Read the model definition and answer for the solid it produces. Units are mm, in the model's axes. Face numbers are marked on the shaded views. A direction names the side the tool comes from. Coordinates: 2 decimals unless noted, no trailing zeros. Write each loop counter-clockwise with the first axis right and the second up, starting at its lowest first coordinate (ties: lowest second). Pieces come first, ordered by that corner, then holes.
(1) Which of the six approach directions +Z, -Z, +X, -X, +Y, -Y give full straight-line access (tool end or side, diameter ignored) to the marked faces 1 and 2?
(2) Find the intervals of material crossed by probe 1 along X at (y, z) = (-26, 20); probe 2 along Y at (x, z) = (-25, 1.25); probe 3 along X at (y, z) = (2.5, 10.5), in increasing order.
(3) Given pin 1 (1.8 mm diameter, centred on y = -30.98, z = 12, fed in from -X); pin 2 (12 mm diameter, centred on x = -17, z = 15.5, fed in from -Y); pin 3 (8 mm diameter, centred on x = -34, z = 14.5, fed in from -Y); pin 4 (10 mm diameter, centred on x = -37, z = 15.5, fed in from -Y), each flat-ended and moving along its own axis, determine where each tip first touches the part or whether it passes through.
(4) Section C-C on z = 10.25 is taken. Write down the section's boundary in (x, y), then the cut area to 3 significant figures.
(5) Section A-A on y = -18 is taken. Write down the section's boundary in (x, z).
(6) Section B-B on z = 15 is taken. Write down the section's boundary in (x, y).
(7) Section D-D on x = -7 is taken. Write down the section's boundary in (y, z).
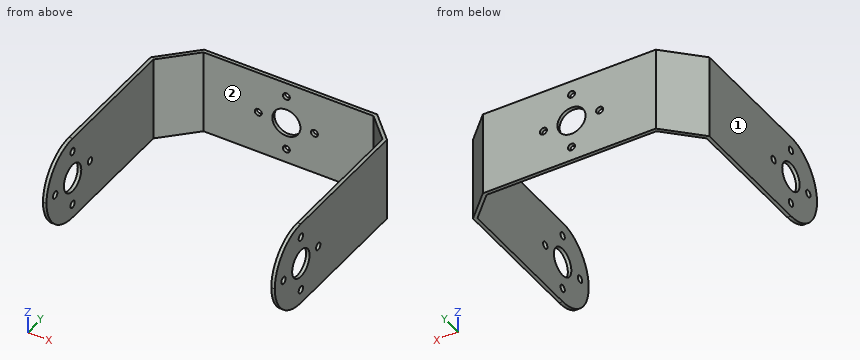
from build123d import *

# Parameters (mm, degrees)
BOSS_EXTRUDE1_DEPTH = 24
SKETCH5_R           = 1
SKETCH5_R_2         = 4
CUT_EXTRUDE3_DEPTH  = 1
CUT_EXTRUDE4_START  = -1
SKETCH6_R           = 4
SKETCH6_R_2         = 1
CUT_EXTRUDE4_DEPTH  = 1
SKETCH7_R           = 4
SKETCH7_R_2         = 1
CUT_EXTRUDE5_DEPTH  = 1
FILLET1_R           = 12


with BuildPart() as part:
    # Sketch1 → Boss-Extrude1 (new body)
    with BuildSketch(Plane.XY):
        Polygon((18.706612688, 0.24678935), (18.706612688, -50.981637775), (19.706612688, -50.981637775), (19.706612688, 0.661002912), (12.349253376, 8.018362225), (-36.879173749, 8.018362225), (-46.293387312, -1.395851338), (-46.293387312, -50.981637775), (-45.293387312, -50.981637775), (-45.293387312, -1.8100649), (-36.464960187, 7.018362225), (11.935039813, 7.018362225), align=None)
    extrude(amount=BOSS_EXTRUDE1_DEPTH)

    # Sketch5 → Cut-Extrude3 (cut)
    with BuildSketch(Plane.ZY.offset(46.293387312)):
        with Locations((20, -38.981637775)):
            Circle(SKETCH5_R)
        with Locations((12, -38.981637775)):
            Circle(SKETCH5_R_2)
        with Locations((12, -46.981637775)):
            Circle(SKETCH5_R)
        with Locations((4, -38.981637775)):
            Circle(SKETCH5_R)
        with Locations((12, -30.981637775)):
            Circle(SKETCH5_R)
    extrude(amount=-CUT_EXTRUDE3_DEPTH, mode=Mode.SUBTRACT)

    # Sketch6 → Cut-Extrude4 (cut)
    with BuildSketch(Plane(origin=(19.706612688, 0, 0), x_dir=(0, 0, -1), z_dir=(1, 0, 0)).offset(CUT_EXTRUDE4_START)):
        with Locations(Location((-12, -38.981637775, 0), (0, 0, 180))):
            Circle(SKETCH6_R)
        with Locations(Location((-4, -38.981637775, 0), (0, 0, 180))):
            Circle(SKETCH6_R_2)
        with Locations(Location((-12, -46.981637775, 0), (0, 0, 180))):
            Circle(SKETCH6_R_2)
        with Locations(Location((-20, -38.981637775, 0), (0, 0, 180))):
            Circle(SKETCH6_R_2)
        with Locations(Location((-12, -30.981637775, 0), (0, 0, 180))):
            Circle(SKETCH6_R_2)
    extrude(amount=CUT_EXTRUDE4_DEPTH, mode=Mode.SUBTRACT)

    # Sketch7 → Cut-Extrude5 (cut)
    with BuildSketch(Plane(origin=(0, 8.018362225, 0), x_dir=(1, 0, 0), z_dir=(0, 1, 0))):
        with Locations(Location((-12.879173749, -12, 0), (0, 0, 180))):
            Circle(SKETCH7_R)
        with Locations(Location((-12.879173749, -20, 0), (0, 0, 180))):
            Circle(SKETCH7_R_2)
        with Locations(Location((-20.879173749, -12, 0), (0, 0, 180))):
            Circle(SKETCH7_R_2)
        with Locations(Location((-12.879173749, -4, 0), (0, 0, 180))):
            Circle(SKETCH7_R_2)
        with Locations(Location((-4.879173749, -12, 0), (0, 0, 180))):
            Circle(SKETCH7_R_2)
    extrude(amount=-CUT_EXTRUDE5_DEPTH, mode=Mode.SUBTRACT)

    # Fillet1
    fillet1_edges = [part.edges().sort_by_distance(p)[0] for p in [
        (19.206612688, -50.981637775, 24),
        (19.206612688, -50.981637775, 0),
        (-45.793387312, -50.981637775, 24),
        (-45.793387312, -50.981637775, 0),
    ]]
    fillet(fillet1_edges, radius=FILLET1_R - 0.0001)  # a hair under: the kernel refuses the full size


solid = part.part
Response:
1. face 1: +Z, -Z, -X, +Y, -Y
1. face 2: +Z, -Z, -Y
2. probe 1: x = -46.29 to -45.29, 18.71 to 19.71
2. probe 2: y = 7.02 to 8.02
2. probe 3: x = -42.4 to -40.98, 16.45 to 17.87
3. pin 1: passes through
3. pin 2: stops at y = 7.02
3. pin 3: stops at y = 5.48
3. pin 4: stops at y = 1.48
4. outline: (-46.29, -50.85) - (-45.29, -50.85) - (-45.29, -42.58) - (-46.29, -42.58) - close; (-46.29, -35.38) - (-45.29, -35.38) - (-45.29, -1.81) - (-36.46, 7.02) - (-16.48, 7.02) - (-16.48, 8.02) - (-36.88, 8.02) - (-46.29, -1.4) - close; (-9.28, 7.02) - (11.94, 7.02) - (18.71, 0.25) - (18.71, -35.38) - (19.71, -35.38) - (19.71, 0.66) - (12.35, 8.02) - (-9.28, 8.02) - close; (18.71, -50.85) - (19.71, -50.85) - (19.71, -42.58) - (18.71, -42.58) - close
4. area: 151 mm2
5. outline: (-46.29, 0) - (-45.29, 0) - (-45.29, 24) - (-46.29, 24) - close; (18.71, 0) - (19.71, 0) - (19.71, 24) - (18.71, 24) - close
6. outline: (-46.29, -50.6) - (-45.29, -50.6) - (-45.29, -41.63) - (-46.29, -41.63) - close; (-46.29, -36.34) - (-45.29, -36.34) - (-45.29, -1.81) - (-36.46, 7.02) - (-15.52, 7.02) - (-15.52, 8.02) - (-36.88, 8.02) - (-46.29, -1.4) - close; (-10.23, 7.02) - (11.94, 7.02) - (18.71, 0.25) - (18.71, -36.34) - (19.71, -36.34) - (19.71, 0.66) - (12.35, 8.02) - (-10.23, 8.02) - close; (18.71, -50.6) - (19.71, -50.6) - (19.71, -41.63) - (18.71, -41.63) - close
7. outline: (7.02, 0) - (8.02, 0) - (8.02, 24) - (7.02, 24) - close
